from build123d import *

# Parameters (mm, degrees)
F0_W     = 25
F0_H     = 17.9
F1_DEPTH = 10
F3_D     = 5
F4_W     = 10
F4_H     = 17.9
F5_DEPTH = 25
F6_R     = 1.66
F7_DEPTH = 25


# Not quite as in the source:
# - a feature names something its author has since deleted; it is built from what else it names


with BuildPart() as f1:
    # F0 (on Front) → F1 (new body)
    with BuildSketch(Plane.XZ):
        Polygon((-11.5858212113, -12.1098860052), (-11.5858212113, 5.7901139948), (-33.1716425717, 3.0010114424), (-32.9104475677, -5.8795856312), align=None)
        with Locations((0.9141787887, -3.1598860052)):
            Rectangle(F0_W, F0_H)
    extrude(amount=F1_DEPTH)

    # F3 (through all)
    with Locations(Plane.XZ.offset(10)):
        with Locations((7.2585181333, 2.1878613625), (7.2585181333, -6.9218412973)):
            Hole(F3_D / 2)

    # F4 (on face) → F5 (join)
    with BuildSketch(Plane.YZ.offset(13.4141787887)):
        with Locations((-5, -3.1598860052)):
            Rectangle(F4_W, F4_H)
    extrude(amount=F5_DEPTH)

    # F6 (on face) → F7 (cut)
    with BuildSketch(Plane.XY.offset(5.7901139948)):
        with Locations((29.4916108251, -4.9681207165)):
            Circle(F6_R)
    extrude(amount=-F7_DEPTH, mode=Mode.SUBTRACT)


solid = f1.part
Design review of the part built by this model. Coordinates are the model's own, in mm. Round coordinates to 2 decimals unless told otherwise and drop trailing zeros. Write each loop counter-clockwise with the first axis right and the second up, starting at its lowest first coordinate (ties: lowest second). Pieces come first, ordered by that corner, then holes. Notation, with made-up numbers: (-39, -32.75) - (-15, -32.75) arc R28 cw to (-15, -1.75) - close; hole circle Ø5 at (-8, 31). An arc over 180 degrees is marked (long way). Use a Markdown table: item, result. Add a question column.
1. Wall thickness on probe 1 along X at (y, z) = (-7.75, 0.5); probe 2 along Z at (x, y) = (9.5, -4.5) (3 decimals); probe 3 along X at (y, z) = (-4.75, -2): over which ranges is each line inside the solid? List them lowest first.
2. We need section D-D (x = -16.5). State the section outline as (y, z) points, then the cut area to 3 significant figures.
3. Mouldability with a two-part tool opening along Y and no side actions: class faces 1 (the face through (-22.228, -4.93, 4.415)), 2 (the face through (30.384, -3.568, -3.035)), 3 (the face through (2, 0, -3)) as +Y half, -Y half, draft (parallel to the pull), parting line (faces both ways), or undercut.
4. We need section B-B (y = -1.25). State the section outline as (x, z) points.
5. We need section C-C (z = 4). State the section outline as (x, y) points, then the cut area to 3 significant figures.
6. Clearance check with flat-ended pins moving along their axes: pin 1 (4 mm diameter, centred on x = 7.26, z = 2.19, fed in from -Y); pin 2 (1 mm diameter, centred on y = -6, z = -4.5, fed in from -X). State where each tip first meets the part, or that it passes through.
7. We need section A-A (z = -8). State the section outline as (x, y) points, then the cut area to 3 significant figures.
Output:
| question | item | result |
|---|---|---|
| 1 | probe 1 | x = -33.1 to 5.41, 9.1 to 38.41 |
| 1 | probe 2 | z = -12.11 to -8.029, -5.815 to 1.081, 3.295 to 5.79 |
| 1 | probe 3 | x = -33.02 to 27.85, 31.14 to 38.41 |
| 2 | outline | (-10, -10.67) - (0, -10.67) - (0, 5.16) - (-10, 5.16) - close |
| 2 | area | 158 mm2 |
| 3 | face 1 | draft |
| 3 | face 2 | undercut |
| 3 | face 3 | +Y half |
| 4 | outline | (-33.17, 3) - (-32.91, -5.88) - (-11.59, -12.11) - (38.41, -12.11) - (38.41, 5.79) - (-11.59, 5.79) - close; hole circle Ø5 at (7.26, -6.92); hole circle Ø5 at (7.26, 2.19) |
| 5 | outline | (-25.44, -10) - (5.54, -10) - (5.54, 0) - (-25.44, 0) - close; (8.98, -10) - (38.41, -10) - (38.41, 0) - (8.98, 0) - close; hole circle Ø3.32 at (29.49, -4.97) |
| 5 | area | 595 mm2 |
| 6 | pin 1 | passes through |
| 6 | pin 2 | stops at x = -32.97 |
| 7 | outline | (-25.65, -10) - (5, -10) - (5, 0) - (-25.65, 0) - close; (9.51, -10) - (38.41, -10) - (38.41, 0) - (9.51, 0) - close; hole circle Ø3.32 at (29.49, -4.97) |
| 7 | area | 587 mm2 |
